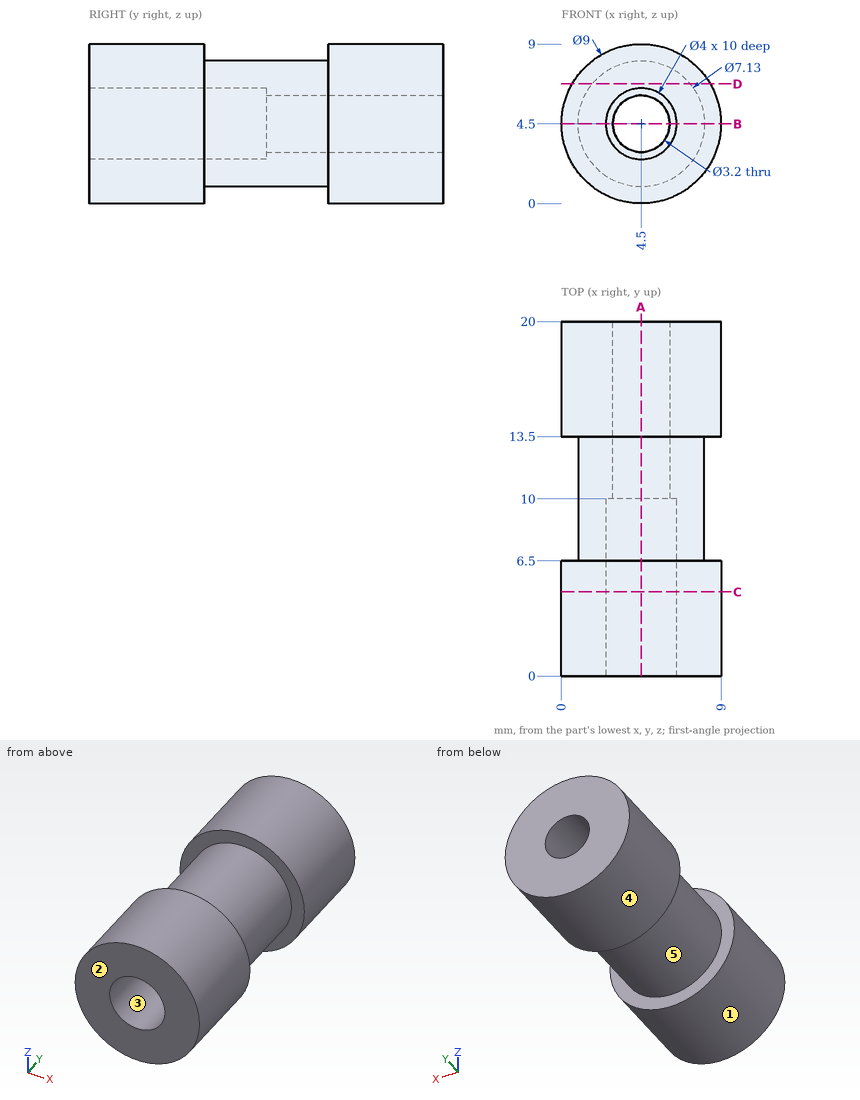
Study the drawing (mm; zero at the part's minimum x, y, z) and answer. A direction names the side the tool comes from. Coordinates: 2 decimals unless noted, no trailing zeros. Write each loop counter-clockwise with the first axis right and the second up, starting at its lowest first coordinate (ties: lowest second). Pieces come first, ordered by that corner, then holes. Notation, with made-up numbers: (32, 52) - (49, 52) arc R16 cw to (49, 64) - close; hole circle Ø7 at (85.5, 87.5). An arc over 180 degrees is marked (long way). Return JSON: item names as keys, results as strings. Group by question number.
1. Which of the six approach directions +Z, -Z, +X, -X, +Y, -Y give full straight-line access (tool end or side, diameter ignored) to the marked faces 4 and 5?
2. Straight lines are drawn through the part: L1, parallel to Z at x = 4.5, y = 17; L2, parallel to Y at x = 5.5, z = 8.5. For each, find the intervals that lie inside material, in ascending order.
3. A cutting plane is placed at B-B, the plane z = 4.5. Determine the outline of the cut face in (x, y) (3 decimals).
4. A cutting plane is placed at D-D, the plane z = 6.75. Determine the outline of the cut face in (x, y).
5. A cutting plane is placed at A-A, the plane x = 4.5. Determine the outline of the cut face in (y, z) (3 decimals), plus the area to 3 significant figures.
6. A cutting plane is placed at C-C, the plane y = 4.75. Determine the outline of the cut face in (x, z).
7. Determine the mould class of the marked faces 1, 2 and 3 for opening direction X: released by +X, released by -X, zero draft, split by the parting line, or undercut.
8. Given pin 1 (2 mm diameter, centred on x = 7, y = 14.5, fed in from +Z), flat-ended and moving along its own axis, determine where the tip first touches the part or whether it passes through.
Ans:
{
 "1": {"face 4": "+Y, -Y", "face 5": "none"},
 "2": {"L1": "0 to 2.9, 6.1 to 9", "L2": "0 to 6.5, 13.5 to 20"},
 "3": {"outline": "(0, 0) - (2.5, 0) - (2.5, 10) - (2.9, 10) - (2.9, 20) - (0, 20) - (0, 13.5) - (0.935, 13.5) - (0.935, 6.5) - (0, 6.5) - close; (6.1, 10) - (6.5, 10) - (6.5, 0) - (9, 0) - (9, 6.5) - (8.065, 6.5) - (8.065, 13.5) - (9, 13.5) - (9, 20) - (6.1, 20) - close"},
 "4": {"outline": "(0.6, 0) - (8.4, 0) - (8.4, 6.5) - (7.27, 6.5) - (7.27, 13.5) - (8.4, 13.5) - (8.4, 20) - (0.6, 20) - (0.6, 13.5) - (1.73, 13.5) - (1.73, 6.5) - (0.6, 6.5) - close"},
 "5": {"outline": "(0, 0) - (6.5, 0) - (6.5, 0.935) - (13.5, 0.935) - (13.5, 0) - (20, 0) - (20, 2.9) - (10, 2.9) - (10, 2.5) - (0, 2.5) - close; (0, 6.5) - (10, 6.5) - (10, 6.1) - (20, 6.1) - (20, 9) - (13.5, 9) - (13.5, 8.065) - (6.5, 8.065) - (6.5, 9) - (0, 9) - close", "area": "94.9 mm²"},
 "6": {"outline": "circle Ø9 at (4.5, 4.5); hole circle Ø4 at (4.5, 4.5)"},
 "7": {"face 1": "split by the parting line", "face 2": "zero draft", "face 3": "undercut"},
 "8": {"pin 1": "z = 8.74"}
}
